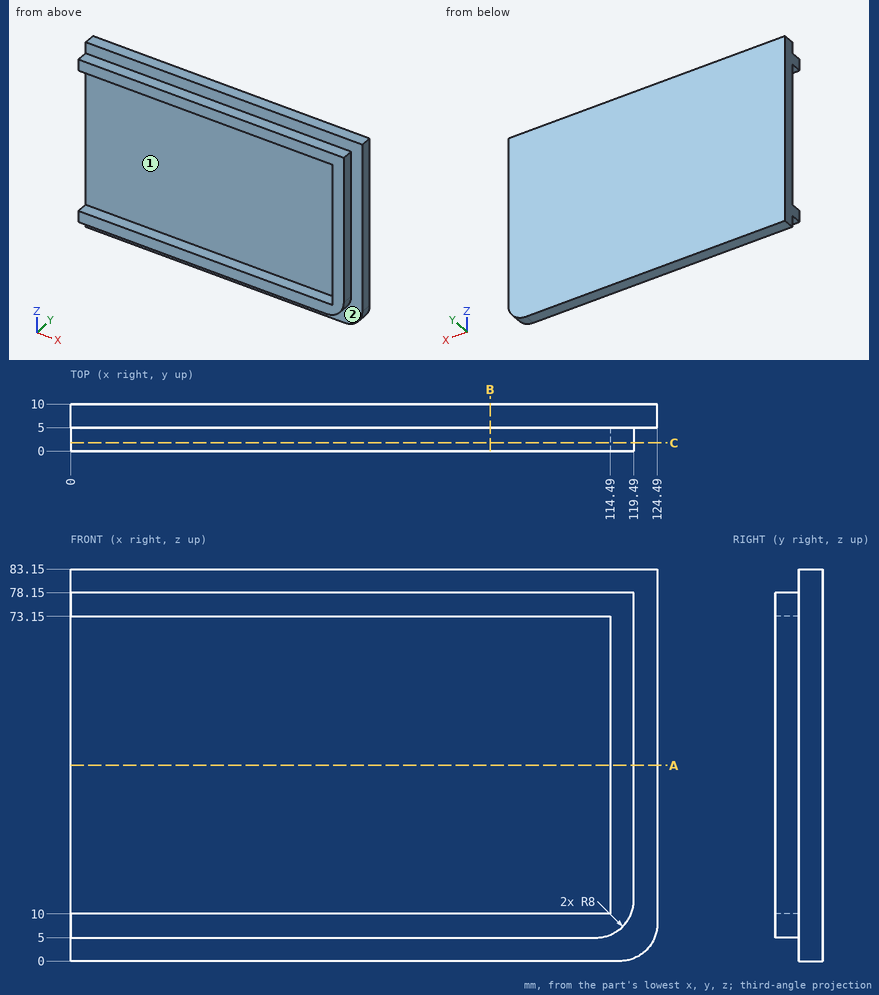
Input: dimensioned drawing with shaded views. Units: mm. Origin: part minimum x, y, z. Coordinates: 2 decimals unless noted, no trailing zeros. Order: outer loops, then holes, each group sorted by start corner. A loop starts at its lowest first (then second) coordinate and runs counter-clockwise, first axis right, second up. Notation, with made-up numbers: (48, -10) - (73, -10) arc R24 ccw to (73, 25) - close; hole circle Ø4 at (75.5, 61.25). An arc over 180 degrees is marked (long way). Return JSON: item names as keys, results as strings. Group by question number.
1. Pull-direction query (Z, two-part tool) for the marked faces 1 and 2; classes: pulls with the +Z half, pulls with the -Z half, needs draft (parallel to the pull), parting line crosses it, or undercut.
2. Pin query (flat end, axial travel): pin 1 (1.5 mm diameter, centred on x = 50, y = 1.5, fed in from +Z); pin 2 (5.5 mm diameter, centred on y = 2, z = 38.5, fed in from +X); pin 3 (2.5 mm diameter, centred on x = 35.5, y = 3, fed in from -Z). Return the tip coordinate at first contact, or that it passes through.
3. Cut plane B-B (x = 89). Output: boundary loops of the cut face in (y, z).
4. Cut plane A-A (z = 41.5). Output: boundary loops of the cut face in (x, y), plus the area to 3 significant figures.
5. Material intervals for line 1 along Z through (x, y) = (56, 0.5); line 2 along Y through (x, z) = (33.5, 38); line 3 along X through (y, z) = (1, 55.5), sorted ascending. Write a range as [from, to].
6. Cut plane C-C (y = 1.75). Output: boundary loops of the cut face in (x, z).
Resolved:
{
 "1": {"face 1": "undercut", "face 2": "needs draft"},
 "2": {"pin 1": "stops at z = 78.15", "pin 2": "stops at x = 119.49", "pin 3": "stops at z = 5"},
 "3": {"outline": "(0, 5) - (5, 5) - (5, 0) - (10, 0) - (10, 83.15) - (5, 83.15) - (5, 78.15) - (0, 78.15) - (0, 73.15) - (5, 73.15) - (5, 10) - (0, 10) - close"},
 "4": {"outline": "(0, 5) - (114.49, 5) - (114.49, 0) - (119.49, 0) - (119.49, 5) - (124.49, 5) - (124.49, 10) - (0, 10) - close", "area": "647 mm²"},
 "5": {"line 1": "z = [5, 10], [73.15, 78.15]", "line 2": "y = [5, 10]", "line 3": "x = [114.49, 119.49]"},
 "6": {"outline": "(0, 5) - (111.49, 5) arc R8 ccw to (119.49, 13) - (119.49, 78.15) - (0, 78.15) - (0, 73.15) - (114.49, 73.15) - (114.49, 10) - (0, 10) - close"}
}
